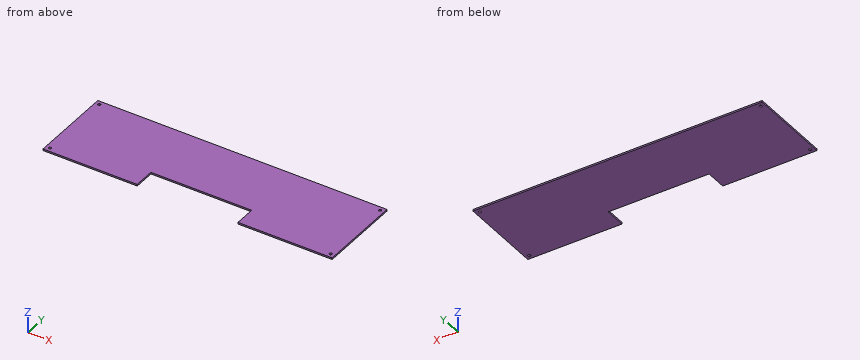
from build123d import *

# Parameters (mm, degrees)
SKETCH_1_W          = 344.5
SKETCH_1_H          = 100
EXTRUDE_1_DEPTH     = 2
SKETCH_2_R          = 1.6
CUT_EXTRUDE_1_DEPTH = 2
SKETCH_3_W          = 120
SKETCH_3_H          = 25
CUT_EXTRUDE_2_DEPTH = 10


with BuildPart() as part:
    # 草图1 → 凸台-拉伸1 (new body)
    with BuildSketch(Plane.XY):
        Rectangle(SKETCH_1_W, SKETCH_1_H)
    extrude(amount=EXTRUDE_1_DEPTH)

    # 草图2 → 切除-拉伸1 (cut)
    with BuildSketch(Plane.XY.offset(2)):
        with Locations((167.25, -45)):
            Circle(SKETCH_2_R)
        with Locations(Location((167.25, 45, 0), (0, 0, 180))):
            Circle(SKETCH_2_R)
        with Locations(Location((-167.25, -45, 0), (0, 0, 180))):
            Circle(SKETCH_2_R)
        with Locations((-167.25, 45)):
            Circle(SKETCH_2_R)
    extrude(amount=-CUT_EXTRUDE_1_DEPTH, mode=Mode.SUBTRACT)

    # 草图3 → 切除-拉伸2 (cut)
    with BuildSketch(Plane.XY.offset(2)):
        with Locations((0, -37.5)):
            Rectangle(SKETCH_3_W, SKETCH_3_H)
    extrude(amount=-CUT_EXTRUDE_2_DEPTH, mode=Mode.SUBTRACT)


solid = part.part
Design review of the part built by this model. Coordinates are the model's own, in mm. Coordinates: 2 decimals unless noted, no trailing zeros. Order: outer loops, then holes, each group sorted by start corner. A loop starts at its lowest first (then second) coordinate and runs counter-clockwise, first axis right, second up. Notation, with made-up numbers: (10, 13) -> (35, 13) arc R27 ccw to (35, 38) -> close; hole circle Ø8 at (65, 4). An arc over 180 degrees is marked (long way). Use one line per item in the form item = value. Start each with the question number.
(1) Insertion check: pin 1 (1 mm diameter, centred on x = -2.5, z = 1.5, fed in from -Y). The pin has a flat end and moves straight along its axis. Give the tip position at first contact, or say it passes through.
(2) Add section A-A on y = -40. State the section outline as (x, z) points, plus the area to 3 significant figures.
(3) Add section C-C on x = 28.5. State the section outline as (y, z) points, plus the area to 3 significant figures.
(4) Add section B-B on z = 0.45. State the section outline as (x, y) points, plus the area to 3 significant figures.
(5) For probe 1 along Y at (x, z) = (167.25, 1.2); probe 2 along X at (y, z) = (-30, 1.75); probe 3 along X at (y, z) = (46, 1.4), list the stretches that pass through material, from the lowest coordinate up.
Answer block:
q1.pin_1 = -25
q2.outline = (-172.25, 0) -> (-60, 0) -> (-60, 2) -> (-172.25, 2) -> close; (60, 0) -> (172.25, 0) -> (172.25, 2) -> (60, 2) -> close
q2.area = 449 mm²
q3.outline = (-25, 0) -> (50, 0) -> (50, 2) -> (-25, 2) -> close
q3.area = 150 mm²
q4.outline = (-172.25, -50) -> (-60, -50) -> (-60, -25) -> (60, -25) -> (60, -50) -> (172.25, -50) -> (172.25, 50) -> (-172.25, 50) -> close; hole circle Ø3.2 at (-167.25, -45); hole circle Ø3.2 at (-167.25, 45); hole circle Ø3.2 at (167.25, -45); hole circle Ø3.2 at (167.25, 45)
q4.area = 31,400 mm²
q5.probe_1 = -50 to -46.6, -43.4 to 43.4, 46.6 to 50
q5.probe_2 = -172.25 to -60, 60 to 172.25
q5.probe_3 = -172.25 to -168.5, -166 to 166, 168.5 to 172.25
